Verification items for the finished model (mm, model axes). Round coordinates to 2 decimals unless told otherwise and drop trailing zeros. Write each loop counter-clockwise with the first axis right and the second up, starting at its lowest first coordinate (ties: lowest second). Pieces come first, ordered by that corner, then holes. Notation, with made-up numbers: (-29.5, 83.25) - (-5.5, 83.25) arc R29 cw to (-5.5, 116.25) - close; hole circle Ø5 at (79, 78). An arc over 180 degrees is marked (long way). Answer as a JSON object with one key per item and string values.
```python
from build123d import *

# Parameters (mm, degrees)
EXTRUDE_1_DEPTH     = 0.5
SKETCH_3_W          = 1
SKETCH_3_H          = 6
CUT_EXTRUDE_1_DEPTH = 0.5


with BuildPart() as part:
    # 草图1 → 凸台-拉伸1 (new body)
    with BuildSketch(Plane.XY):
        Polygon((-4.5, 0), (-4.5, 67.5), (4.5, 67.5), (4.5, 0), (10, 0), (10, 78), (-10, 78), (-10, 0), align=None)
    extrude(amount=EXTRUDE_1_DEPTH)

    # 草图3 → 切除-拉伸1 (cut)
    with BuildSketch(Plane.XY.offset(0.5)):
        with Locations((-7.5, 74)):
            Rectangle(SKETCH_3_W, SKETCH_3_H)
        with Locations((-4.5, 74)):
            Rectangle(SKETCH_3_W, SKETCH_3_H)
        with Locations((-1.5, 74)):
            Rectangle(SKETCH_3_W, SKETCH_3_H)
        with Locations((1.5, 74)):
            Rectangle(SKETCH_3_W, SKETCH_3_H)
        with Locations((4.5, 74)):
            Rectangle(SKETCH_3_W, SKETCH_3_H)
        with Locations((7.5, 74)):
            Rectangle(SKETCH_3_W, SKETCH_3_H)
        with Locations((-7.5, 64)):
            Rectangle(SKETCH_3_W, SKETCH_3_H)
        with Locations((7.5, 64)):
            Rectangle(SKETCH_3_W, SKETCH_3_H)
        with Locations((-7.5, 54)):
            Rectangle(SKETCH_3_W, SKETCH_3_H)
        with Locations((7.5, 54)):
            Rectangle(SKETCH_3_W, SKETCH_3_H)
        with Locations((-7.5, 44)):
            Rectangle(SKETCH_3_W, SKETCH_3_H)
        with Locations((7.5, 44)):
            Rectangle(SKETCH_3_W, SKETCH_3_H)
        with Locations((-7.5, 34)):
            Rectangle(SKETCH_3_W, SKETCH_3_H)
        with Locations((7.5, 34)):
            Rectangle(SKETCH_3_W, SKETCH_3_H)
        with Locations((-7.5, 24)):
            Rectangle(SKETCH_3_W, SKETCH_3_H)
        with Locations((7.5, 24)):
            Rectangle(SKETCH_3_W, SKETCH_3_H)
        with Locations((-7.5, 14)):
            Rectangle(SKETCH_3_W, SKETCH_3_H)
        with Locations((7.5, 14)):
            Rectangle(SKETCH_3_W, SKETCH_3_H)
        with Locations((-7.5, 4)):
            Rectangle(SKETCH_3_W, SKETCH_3_H)
        with Locations((7.5, 4)):
            Rectangle(SKETCH_3_W, SKETCH_3_H)
    extrude(amount=-CUT_EXTRUDE_1_DEPTH, mode=Mode.SUBTRACT)


solid = part.part
```
1. Cross-section at A-A (y = 43). Record the boundary of the cut face in (x, z), plus the area to 3 significant figures.
Completed:
{"outline": "(-10, 0) - (-8, 0) - (-8, 0.5) - (-10, 0.5) - close; (-7, 0) - (-4.5, 0) - (-4.5, 0.5) - (-7, 0.5) - close; (4.5, 0) - (7, 0) - (7, 0.5) - (4.5, 0.5) - close; (8, 0) - (10, 0) - (10, 0.5) - (8, 0.5) - close", "area": "4.50 mm^2"}
2. Cross-section at B-B (z = 0.1). Count the separate pieces of the cut face and the enclosed holes in it, plus the area to 4 significant figures.
Completed:
{"separate pieces": "1", "enclosed holes": "20", "area": "832.5 mm^2"}
3. Cross-section at C-C (x = -0.25). Record the boundary of the cut face in (y, z), plus the area to 3 significant figures.
Completed:
{"outline": "(67.5, 0) - (78, 0) - (78, 0.5) - (67.5, 0.5) - close", "area": "5.25 mm^2"}
4. Material ranges on probe 1 along X at (y, z) = (65, 0.4); probe 2 along X at (y, z) = (8, 0.1); probe 3 along Y at (x, z) = (1.25, 0.2), recorded low to high. Write a range as from..to.
Completed:
{"probe 1": "x = -10..-8, -7..-4.5, 4.5..7, 8..10", "probe 2": "x = -10..-4.5, 4.5..10", "probe 3": "y = 67.5..71, 77..78"}
